Verification items for this drawing (mm, ordinates from the low corner). A direction names the side the tool comes from. Round coordinates to 2 decimals unless told otherwise and drop trailing zeros. Write each loop counter-clockwise with the first axis right and the second up, starting at its lowest first coordinate (ties: lowest second). Pieces come first, ordered by that corner, then holes. Notation, with made-up numbers: (-12.5, -6.75) -> (16.5, -6.75) arc R11 ccw to (16.5, -0.75) -> close; hole circle Ø11 at (-13, -8.5). An arc over 180 degrees is marked (long way). One line per question, with ' | ' between items.
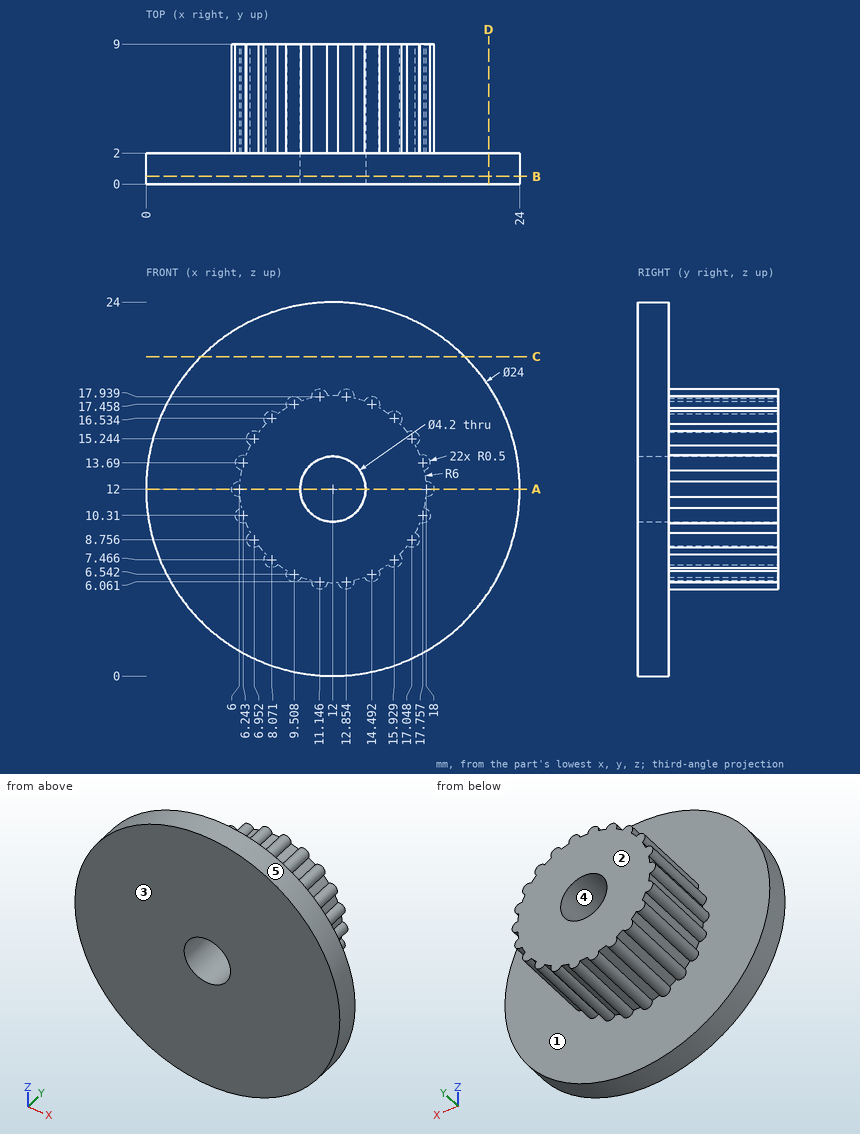
(1) Sectioned sample at A-A on z = 12. Record the cut outline in (x, y).
Resolved:
outline: (0, 0) -> (9.9, 0) -> (9.9, 9) -> (5.5, 9) -> (5.5, 2) -> (0, 2) -> close; (14.1, 0) -> (24, 0) -> (24, 2) -> (18.5, 2) -> (18.5, 9) -> (14.1, 9) -> close
(2) Go/stop test with flat-tipped pins: pin 1 (3 mm diameter, centred on x = 3.5, y = 8, fed in from -Z); pin 2 (6.5 mm diameter, centred on x = 12, z = 12, fed in from -Y); pin 3 (3 mm diameter, centred on x = 6.5, y = 4, fed in from +Z); pin 4 (4 mm diameter, centred on x = 19, y = 7.5, fed in from +Z). Record where each tip stops, or that it passes through.
Resolved:
pin 1: passes through | pin 2: stops at y = 0 | pin 3: stops at z = 17.03 | pin 4: stops at z = 15.74
(3) Sectioned sample at C-C on z = 20.5. Record the cut outline in (x, y).
Resolved:
outline: (3.53, 0) -> (20.47, 0) -> (20.47, 2) -> (3.53, 2) -> close
(4) Material ranges on line 1 (Z direction, x = 12, y = 6); line 2 (X direction, y = 3, z = 12); line 3 (Y direction, x = 6.25, z = 22), recorded low to high.
Resolved:
line 1: z = 6 to 9.9, 14.1 to 18 | line 2: x = 5.5 to 9.9, 14.1 to 18.5 | line 3: y = 0 to 2
(5) Sectioned sample at B-B on y = 0.5. Record the cut outline in (x, z).
Resolved:
outline: circle Ø24 at (12, 12); hole circle Ø4.2 at (12, 12)
(6) Draft check along X on the marked faces 3, 4 and 5. Enter one of: +X half, -X half, draft (parallel to the pull), parting line (faces both ways), or undercut.
Resolved:
face 3: draft | face 4: undercut | face 5: parting line
(7) Sectioned sample at D-D on x = 22. Record the cut outline in (y, z).
Resolved:
outline: (0, 5.37) -> (2, 5.37) -> (2, 18.63) -> (0, 18.63) -> close
(8) Access from +Z, -Z, +X, -X, +Y, -Y to the whole of each face (thin tool, end or side, straight path). Record for the marked faces 1 and 2.
Resolved:
face 1: +Y | face 2: +Z, -Z, +X, -X, +Y
